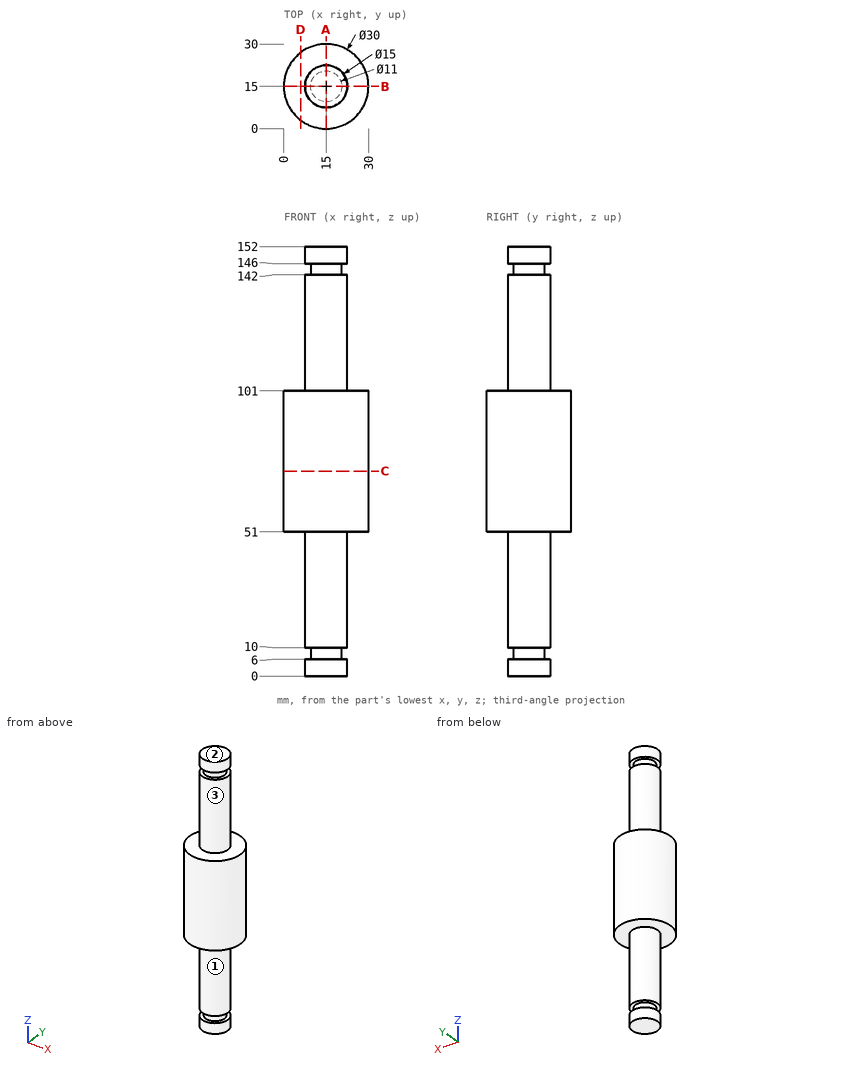
Can you work these out from the drawing? Everything is in mm from the part's minimum corner. A direction names the side the tool comes from. Coordinates: 2 decimals unless noted, no trailing zeros. Loops run counter-clockwise (first coordinate to the right, second up) from the corner with the lowest first, then second, coordinate; pieces in that order, holes last.
1. Imagine slicing it at A-A, the plane x = 15. Please give me the cut outline in (y, z), and give its area (3 significant figures).
2. Imagine slicing it at C-C, the plane z = 72.5. Please give me the cut outline in (x, y), and give its area (3 significant figures).
3. For the marked faces 1, 2 and 3, which set-ups out of +Z, -Z, +X, -X, +Y, -Y let a thin tool reach every point of the face, with its end or its side?
4. For P1, Ø1.5, axis at x = 5.5, y = 8.5, coming from the +Z side; P2, Ø8, axis at x = 18, z = 119, coming from the -Y side; P3, Ø12, axis at y = 13, z = 19, coming from the +X side, each with a flat end and sliding along its axis, tell me the tip position at first contact or that it passes through.
5. Imagine slicing it at D-D, the plane x = 6. Please give me the cut outline in (y, z), and give its area (3 significant figures).
6. I need wall thicknesses on L1, parallel to Z at x = 22.75, y = 2.5; L2, parallel to X at y = 15.25, z = 131.5; L3, parallel to X at y = 25.25, z = 70.5. Which ranges of each line are inside material? Lowest first, please.
Taken from the geometry:
1. outline: (0, 51) - (7.5, 51) - (7.5, 10) - (9.5, 10) - (9.5, 6) - (7.5, 6) - (7.5, 0) - (22.5, 0) - (22.5, 6) - (20.5, 6) - (20.5, 10) - (22.5, 10) - (22.5, 51) - (30, 51) - (30, 101) - (22.5, 101) - (22.5, 142) - (20.5, 142) - (20.5, 146) - (22.5, 146) - (22.5, 152) - (7.5, 152) - (7.5, 146) - (9.5, 146) - (9.5, 142) - (7.5, 142) - (7.5, 101) - (0, 101) - close
1. area: 3,000 mm2
2. outline: circle Ø30 at (15, 15)
2. area: 707 mm2
3. face 1: -Z
3. face 2: +Z, +X, -X, +Y, -Y
3. face 3: +Z
4. P1: stops at z = 101
4. P2: stops at y = 7.5
4. P3: stops at x = 22.5
5. outline: (3, 51) - (27, 51) - (27, 101) - (3, 101) - close
5. area: 1,200 mm2
6. L1: z = 51 to 101
6. L2: x = 7.5 to 22.5
6. L3: x = 4.05 to 25.95
